from build123d import *

# Parameters (mm, degrees)
IZIM1_W                       = 17
IZIM1_H                       = 34
Y_KSEKLIK_EKSTR_ZYON1_DEPTH   = 1
IZIM2_R                       = 2.5
IZIM2_R_2                     = 1.75
Y_KSEKLIK_EKSTR_ZYON2_DEPTH   = 2
Y_KSEKLIK_EKSTR_ZYON2_2_DEPTH = 2
IZIM3_W                       = 6.690686046
IZIM3_H                       = 5.888560339
IZIM3_W_2                     = 6.077595292
Y_KSEKLIK_EKSTR_ZYON3_DEPTH   = 11


with BuildPart() as part:
    # izim1 → Y_kseklik-Ekstr_zyon1 (new body)
    with BuildSketch(Plane(origin=(0, 0, 0), x_dir=(1, 0, 0), z_dir=(0, 1, 0))):
        Rectangle(IZIM1_W, IZIM1_H)
    extrude(amount=Y_KSEKLIK_EKSTR_ZYON1_DEPTH)



with BuildPart() as body_2:
    # izim2 → Y_kseklik-Ekstr_zyon2 (new body)
    with BuildSketch(Plane.XY.offset(17)):
        with Locations((-4.5, 4)):
            Circle(IZIM2_R)
        with Locations((-4.5, 4)):
            Circle(IZIM2_R_2, mode=Mode.SUBTRACT)
    extrude(amount=Y_KSEKLIK_EKSTR_ZYON2_DEPTH)


with BuildPart() as body_3:
    # izim2 → Y_kseklik-Ekstr_zyon2 2 (new body)
    with BuildSketch(Plane.XY.offset(17)):
        with Locations((4.5, 4)):
            Circle(IZIM2_R)
        with Locations((4.5, 4)):
            Circle(IZIM2_R_2, mode=Mode.SUBTRACT)
    extrude(amount=Y_KSEKLIK_EKSTR_ZYON2_2_DEPTH)


with BuildPart() as part_1:
    add(part.part)

    add(body_2.part)  # Y_kseklik-Ekstr_zyon3 merges body 2

    add(body_3.part)  # Y_kseklik-Ekstr_zyon3 merges body 3
    # izim3 → Y_kseklik-Ekstr_zyon3 (add)
    with BuildSketch(Plane.XY.offset(17)):
        with Locations((-4.46490005, 3.94428017)):
            Rectangle(IZIM3_W, IZIM3_H)
        with Locations((4.558196469, 3.94428017)):
            Rectangle(IZIM3_W_2, IZIM3_H)
    extrude(amount=-Y_KSEKLIK_EKSTR_ZYON3_DEPTH)


solid = part_1.part
The listing builds one solid part. Answer for the finished solid, in the listing's coordinates (mm). A direction names the side the tool comes from. Coordinates: 2 decimals unless noted, no trailing zeros. Loops run counter-clockwise (first coordinate to the right, second up) from the corner with the lowest first, then second, coordinate; pieces in that order, holes last. Notation, with made-up numbers: M 89.5,87 L 110.5,87 A31 ccw 110.5,124 Z; hole C -5,60 d8. An arc over 180 degrees is marked long. Answer in a Markdown table with one row per item.
1) Given pin 1 (4 mm diameter, centred on x = -6, y = 1.5, fed in from -Z); pin 2 (1.5 mm diameter, centred on x = 6, z = -3, fed in from +Y); pin 3 (2 mm diameter, centred on x = 1.5, y = 2, fed in from +Z); pin 4 (4 mm diameter, centred on x = -4.5, y = 4, fed in from -Z), each flat-ended and moving along its own axis, determine where each tip first touches the part or whether it passes through.
Answers below:
| item | result |
|---|---|
| pin 1 | z = -17 |
| pin 2 | y = 1 |
| pin 3 | z = 17 |
| pin 4 | z = 6 |
2) Find section B-B (z = 13.5). Determine the outline of the cut face in (x, y), then the cut area to 3 significant figures.
Answers below:
| item | result |
|---|---|
| outline | M -8.5,0 L 8.5,0 L 8.5,1 L 7.6,1 L 7.6,6.89 L 1.52,6.89 L 1.52,1 L -1.12,1 L -1.12,6.89 L -7.81,6.89 L -7.81,1 L -8.5,1 Z |
| area | 92.2 mm^2 |
3) Determine the mould class of faces 5 (the flat face through (-0.1, 0.5, -17)), 6 (the flat face through (-5, 4, 17)), 7 (the flat face through (-7.81, 4, 12)) for opening direction X: released by +X, released by -X, zero draft, split by the parting line, or undercut.
Answers below:
| item | result |
|---|---|
| face 5 | zero draft |
| face 6 | undercut |
| face 7 | released by -X |
4) Find section A-A (y = 4). Determine the outline of the cut face in (x, z), then the cut area to 3 significant figures.
Answers below:
| item | result |
|---|---|
| outline | M -7.81,6 L -1.12,6 L -1.12,17 L -2,17 L -2,19 L -2.75,19 L -2.75,17 L -6.25,17 L -6.25,19 L -7,19 L -7,17 L -7.81,17 Z; M 1.52,6 L 7.6,6 L 7.6,17 L 7,17 L 7,19 L 6.25,19 L 6.25,17 L 2.75,17 L 2.75,19 L 2,19 L 2,17 L 1.52,17 Z |
| area | 146 mm^2 |
5) Find section D-D (z = -9.5). Determine the outline of the cut face in (x, y), then the cut area to 3 significant figures.
Answers below:
| item | result |
|---|---|
| outline | M -8.5,0 L 8.5,0 L 8.5,1 L -8.5,1 Z |
| area | 17.0 mm^2 |
6) Find the intervals of material crossed by probe 1 along X at (y, z) = (5, 10.5); probe 2 along Y at (x, z) = (-4.5, 18.3); probe 3 along Z at (x, y) = (3.25, 3.75), in increasing order.
Answers below:
| item | result |
|---|---|
| probe 1 | -7.81 to -1.12, 1.52 to 7.6 |
| probe 2 | 1.5 to 2.25, 5.75 to 6.5 |
| probe 3 | 6 to 17 |
7) Find section C-C (x = -4.5). Determine the outline of the cut face in (y, z), then the cut area to 3 significant figures.
Answers below:
| item | result |
|---|---|
| outline | M 0,-17 L 1,-17 L 1,6 L 6.89,6 L 6.89,17 L 6.5,17 L 6.5,19 L 5.75,19 L 5.75,17 L 2.25,17 L 2.25,19 L 1.5,19 L 1.5,17 L 0,17 Z |
| area | 102 mm^2 |
8) Which of the six approach directions +Z, -Z, +X, -X, +Y, -Y give full straight-line access (tool end or side, diameter ignored) to faces 1 (the cylindrical face through (6.885, 4.751, 17.986)), 2 (the flat face through (7.597, 4, 12)), 3 (the flat face through (-1.12, 4, 12)), 4 (the flat face through (-5, 4, 6))?
Answers below:
| item | result |
|---|---|
| face 1 | +Z |
| face 2 | +Z, -Z, +X, +Y |
| face 3 | +Z, -Z, +Y |
| face 4 | -Z, +X, -X, +Y |
